from build123d import *

# Parameters (mm, degrees)
F0_R     = 2.5
F1_DEPTH = 15
F2_R     = 5
F4_DEPTH = 5
F5_DEPTH = 2.5


with BuildPart() as f1:
    # F0 (on Front) → F1 (new body)
    with BuildSketch(Plane.XZ):
        with BuildLine():
            Line((-20.85, 20.85), (-20.85, 0))
            Line((-20.85, 0), (-20.85, -20.85))
            Line((-20.85, -20.85), (0, -20.85))
            Line((0, -20.85), (20.85, -20.85))
            Line((20.85, -20.85), (20.85, 0))
            Line((20.85, 0), (20.85, 20.85))
            Line((20.85, 20.85), (10.425, 20.85))
            Line((10.425, 20.85), (10.425, 47.277337854))
            ThreePointArc((10.425, 47.277337854), (24.8578784585, 67.3380686447), (15, 90))
            Line((15, 90), (15, 110))
            Line((15, 110), (5, 110))
            Line((5, 110), (5, 84.1421356237))
            ThreePointArc((5, 84.1421356237), (14.9999953406, 69.9881770745), (4.9777002722, 55.85))
            Line((4.9777002722, 55.85), (-10.425, 55.85))
            Line((-10.425, 55.85), (-10.425, 20.85))
            Line((-10.425, 20.85), (-20.85, 20.85))
        make_face()
        Polygon((-12.85, 12.85), (0, 12.85), (12.85, 12.85), (12.85, 0), (12.85, -12.85), (0, -12.85), (-12.85, -12.85), (-12.85, 0), align=None, mode=Mode.SUBTRACT)
        with Locations((-5.425, 50.85)):
            Circle(F0_R, mode=Mode.SUBTRACT)
    extrude(amount=F1_DEPTH)

    # F2
    f2_edges = [f1.edges().sort_by_distance(p)[0] for p in [
        (-10.425, -7.5, 55.85),
    ]]
    fillet(f2_edges, radius=F2_R)

    # F3 (on face) → F4 (cut)
    with BuildSketch(Plane.XZ.offset(15)):
        with BuildLine():
            Line((-0.425, 55.85), (-5.425, 55.85))
            ThreePointArc((-5.425, 55.85), (-8.9605339059, 54.3855339059), (-10.425, 50.85))
            Line((-10.425, 50.85), (-10.425, 45.85))
            Line((-10.425, 45.85), (-5.425, 45.85))
            ThreePointArc((-5.425, 45.85), (-1.8894660941, 47.3144660941), (-0.425, 50.85))
            Line((-0.425, 50.85), (-0.425, 55.85))
        make_face()
    extrude(amount=-F4_DEPTH, mode=Mode.SUBTRACT)

    # F5 (add): a face of the model
    f5_faces = [f1.faces().sort_by_distance(p)[0] for p in [
        (4.1569852553, -15, 31.7276341026),
    ]]
    extrude(f5_faces, amount=F5_DEPTH)

    # F7: F1 across plane


with BuildPart() as f1_1:
    add(f1.part)
    add(f1.part.mirror(Plane.XZ.offset(17.5)))


solid = f1_1.part
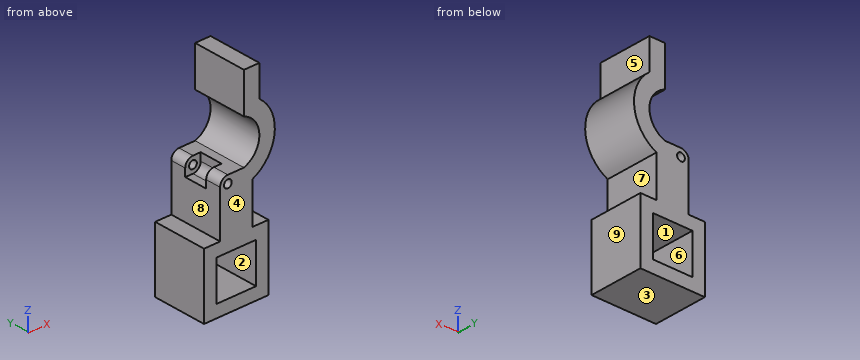
Could you check a few things on this model? Use its own coordinates, in mm. Face numbers are marked on the shaded views. A direction names the side the tool comes from. Give positions to 0.01 mm unless a question says otherwise; leave off trailing zeros. Loops run counter-clockwise (first coordinate to the right, second up) from the corner with the lowest first, then second, coordinate; pieces in that order, holes last. Notation, with made-up numbers: (11, 27.25) -> (16, 27.25) arc R19 cw to (16, 57.25) -> close; hole circle Ø7 at (75, 28.25). An arc over 180 degrees is marked (long way). Answer as CSV lines item,"result". Start each with the question number.
(1) I'm going to push flat-ended pins straight in: pin 1 Ø2.5 at (x, y) = (-7.5, -21) entering from +Z; pin 2 Ø5 at (x, y) = (-13.5, -24.5) entering from +Z; pin 3 Ø1 at (y, z) = (-14.5, 3) entering from +X. Where does each tip first touch, or does it pass through?
(2) I need wall thicknesses on probe 1 along Z at (x, y) = (-2, -6); probe 2 along X at (y, z) = (-33, 11.5); probe 3 along Z at (x, y) = (10, -26.5). Which ranges of each line are inside material? Lowest first, please.
(3) If we section it at B-B on y = -2.5: Write out the boundary of the cut face in (x, z) (3 decimals), then the cut area to 3 significant figures.
(4) Which directions (+Z, -Z, +X, -X, +Y, -Y) give clear straight access to the entire face, cutting with the end or side of a thin tool? Please do the marked faces 5, 6, 7, 8 and 9.
(5) If we section it at D-D on z = 43: Write out the boundary of the cut face in (x, y) (3 decimals), then the cut area to 3 significant figures.
(6) If we section it at A-A on y = -13: Write out the boundary of the cut face in (x, z) (3 decimals), then the cut area to 3 significant figures.
(7) We'd pull the mould along Z, two halves only. Please class the marked faces 1, 2, 3 and 4: released by +Z, released by -Z, zero draft, split by the parting line, or undercut.
(8) If we section it at C-C on z = 16: Write out the boundary of the cut face in (x, y), then the cut area to 3 significant figures.
Computed:
1,pin 1,"stops at z = 45.85"
1,pin 2,"stops at z = 20.85"
1,pin 3,"stops at x = 20.85"
2,probe 1,"z = -20.85 to -12.85, 12.85 to 55.85"
2,probe 2,"x = -20.85 to -12.85, 12.85 to 20.85"
2,probe 3,"z = -20.85 to -12.85, 12.85 to 58.82, 81.18 to 110"
3,outline,"(-20.85, -20.85) -> (20.85, -20.85) -> (20.85, 20.85) -> (10.425, 20.85) -> (10.425, 47.277) arc R25 ccw to (15, 90) -> (15, 110) -> (5, 110) -> (5, 84.142) arc R15 cw to (4.978, 55.85) -> (-5.425, 55.85) arc R5 ccw to (-10.425, 50.85) -> (-10.425, 20.85) -> (-20.85, 20.85) -> close; hole (-12.85, -12.85) -> (12.85, -12.85) -> (12.85, 12.85) -> (-12.85, 12.85) -> close; hole circle Ø5 at (-5.425, 50.85)"
3,area,"2,430 mm2"
4,face 5,"+Z, +X, +Y, -Y"
4,face 6,"+Y, -Y"
4,face 7,"+X, +Y, -Y"
4,face 8,"+Z, -X, +Y, -Y"
4,face 9,"-Z, +X, +Y, -Y"
5,outline,"(-10.425, -35) -> (10.425, -35) -> (10.425, 0) -> (-10.425, 0) -> close"
5,area,"730 mm2"
6,outline,"(-20.85, -20.85) -> (20.85, -20.85) -> (20.85, 20.85) -> (10.425, 20.85) -> (10.425, 47.277) arc R25 ccw to (15, 90) -> (15, 110) -> (5, 110) -> (5, 84.142) arc R15 cw to (4.978, 55.85) -> (-0.425, 55.85) -> (-0.425, 50.85) arc R5 cw to (-5.425, 45.85) -> (-10.425, 45.85) -> (-10.425, 20.85) -> (-20.85, 20.85) -> close; hole (-12.85, -12.85) -> (12.85, -12.85) -> (12.85, 12.85) -> (-12.85, 12.85) -> close"
6,area,"2,360 mm2"
7,face 1,"undercut"
7,face 2,"undercut"
7,face 3,"released by -Z"
7,face 4,"zero draft"
8,outline,"(-20.85, -35) -> (20.85, -35) -> (20.85, 0) -> (-20.85, 0) -> close"
8,area,"1,460 mm2"
